For this review, take the finished solid that the model builds, in its own axes (mm). Face numbers are marked on the shaded views. A direction names the side the tool comes from. Round coordinates to 2 decimals unless told otherwise and drop trailing zeros. Write each loop counter-clockwise with the first axis right and the second up, starting at its lowest first coordinate (ties: lowest second). Pieces come first, ordered by that corner, then holes. Notation, with made-up numbers: (49, -39) -> (54, -39) arc R28 ccw to (54, -15) -> close; hole circle Ø8 at (71, 12.5). An arc over 180 degrees is marked (long way). Write each question's results on one line, items separated by ' | '. Start each with the question number.
Item 1: Add section A-A (y = 11). State the section outline as (x, z) points (3 decimals).
Item 2: Add section B-B (y = -20.5). State the section outline as (x, z) points, plus the area to 3 significant figures.
Item 3: To check wall thickness, follow line 1 along Y through (x, z) = (-8.5, 8.5) (1 decimal); line 2 along Y through (x, z) = (-9.75, 6.75) (3 decimals); line 3 along Y through (x, z) = (-3.75, -9.5) (3 decimals). State the ranges of each line that lie inside material, in increasing order.
Item 4: Clearance check with flat-ended pins moving along their axes: pin 1 (10 mm diameter, centred on y = -50.5, z = -7.5, fed in from +X); pin 2 (12 mm diameter, centred on y = 62, z = -10, fed in from -X); pin 3 (10 mm diameter, centred on x = 0.5, y = -55, fed in from +Z). State where each tip first meets the part, or that it passes through.
Item 5: Tool access review of the marked faces 1 and 2: name each direction out of +Z, -Z, +X, -X, +Y, -Y from which nothing blocks a thin tool from reaching the whole face with its end or side.
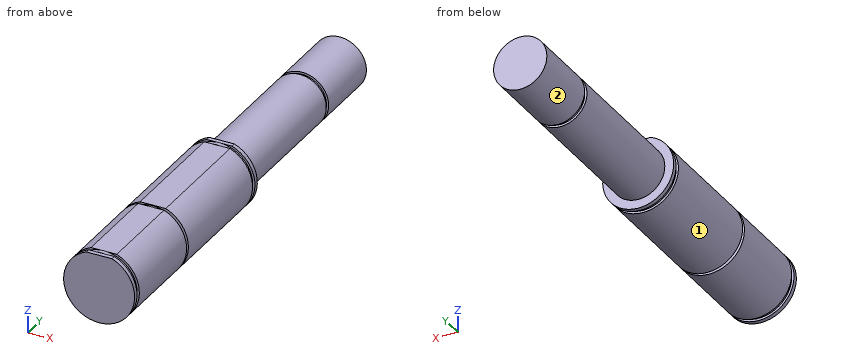
from build123d import *

# Parameters (mm, degrees)
F1_DEPTH  = 76.2
F2_R      = 11.90625
F3_DEPTH  = 1.5875
F5_DEPTH  = 1.5875
F6_R      = 11.90625
F7_DEPTH  = 1.5875
F9_DEPTH  = 1.5875
F10_R     = 9.525
F11_DEPTH = 52.3875
F12_R     = 8.73125
F13_DEPTH = 1.5875
F14_R     = 9.525
F15_DEPTH = 25.4
F16_W     = 1.190625
F16_H     = 1.190625


with BuildPart() as f1:
    # F0 (on Front) → F1 (new body)
    with BuildSketch(Plane.XZ):
        with BuildLine():
            Line((4.6062404769, 11.83522491), (-4.6062404769, 11.83522491))
            ThreePointArc((-4.6062404769, 11.83522491), (0, -12.7), (4.6062404769, 11.83522491))
        make_face()
    extrude(amount=F1_DEPTH)

    # F2 (on face) → F3 (join)
    with BuildSketch(Plane.XZ.offset(76.2)):
        Circle(F2_R)
    extrude(amount=F3_DEPTH)

    # F4 (on face) → F5 (join)
    with BuildSketch(Plane.XZ.offset(77.7875)):
        with BuildLine():
            Line((4.6117921338, 11.8330627191), (-4.6117921338, 11.8330627191))
            ThreePointArc((-4.6117921338, 11.8330627191), (0, -12.7), (4.6117921338, 11.8330627191))
        make_face()
    extrude(amount=F5_DEPTH)

    # F6 (on face) → F7 (join)
    with BuildSketch(Plane(origin=(0, 0, 0), x_dir=(-1, 0, 0), z_dir=(0, 1, 0))):
        Circle(F6_R)
    extrude(amount=F7_DEPTH)

    # F8 (on face) → F9 (join)
    with BuildSketch(Plane(origin=(0, 1.5875, 0), x_dir=(-1, 0, 0), z_dir=(0, 1, 0))):
        with BuildLine():
            Line((4.5204102672, 11.8682724529), (-4.5204102672, 11.8682724529))
            ThreePointArc((-4.5204102672, 11.8682724529), (0, -12.7), (4.5204102672, 11.8682724529))
        make_face()
    extrude(amount=F9_DEPTH)

    # F10 (on face) → F11 (join)
    with BuildSketch(Plane(origin=(0, 3.175, 0), x_dir=(-1, 0, 0), z_dir=(0, 1, 0))):
        Circle(F10_R)
    extrude(amount=F11_DEPTH)

    # F12 (on face) → F13 (join)
    with BuildSketch(Plane(origin=(0, 55.5625, 0), x_dir=(-1, 0, 0), z_dir=(0, 1, 0))):
        Circle(F12_R)
    extrude(amount=F13_DEPTH)

    # F14 (on face) → F15 (join)
    with BuildSketch(Plane(origin=(0, 57.15, 0), x_dir=(-1, 0, 0), z_dir=(0, 1, 0))):
        Circle(F14_R)
    extrude(amount=F15_DEPTH)

    # F16 (on Right) → F17 (revolve, cut)
    with BuildSketch(Plane.YZ):
        with Locations((-43.8153046727, -12.1969180837)):
            Rectangle(F16_W, F16_H)
    revolve(axis=Axis((0, 0, 0), (0, 1, 0)), mode=Mode.SUBTRACT)


solid = f1.part
Responses:
1) outline: circle Ø19.05 at (0, 0)
2) outline: (-4.61, 11.84) arc R12.7 ccw (long way) to (4.61, 11.84) -> close | area: 501 mm^2
3) line 1: y = -79.4 to -77.8, -76.2 to -44.4, -43.2 to 0, 1.6 to 3.2 | line 2: y = -79.375 to -44.411, -43.22 to 3.175 | line 3: y = -79.375 to 3.175
4) pin 1: stops at x = 12.45 | pin 2: stops at x = -8.64 | pin 3: stops at z = 11.84
5) face 1: +Y, -Y | face 2: +Y
